Part model, mm, in its own coordinate system. Coordinates: 2 decimals unless noted, no trailing zeros. Loops run counter-clockwise (first coordinate to the right, second up) from the corner with the lowest first, then second, coordinate; pieces in that order, holes last. Notation, with made-up numbers: (64.25, 6) -> (121.25, 6) arc R32 cw to (121.25, 32) -> close; hole circle Ø7 at (69.5, 79.5). An arc over 180 degrees is marked (long way). Use one line per item in the form item = value. Start each with the question number.
(1) Band-saw the part on B-B on x = -126.5. Give the cut face in (y, z), then the cut area to 4 significant figures.
(2) Band-saw the part on A-A on y = -0.6. Give the cut face in (x, z).
(3) Drill centre line: L1, parallel to Z at x = 372.5, y = -0.9. Where is it in solid material? Low to high. Write a range as [from, to].
(4) Pin check, flat tips, straight feed: P1, Ø12, axis at x = -527, z = -2, coming from the +Y side; P2, Ø1.6, axis at x = -306, y = -0.5, coming from the +Z side; P3, Ø1.5, axis at x = -113.5, z = 27.5, coming from the +Y side. Stop position of each tip, or through.
```python
from build123d import *

# Parameters (mm, degrees)
F0_W     = 1380
F0_H     = 60
F1_DEPTH = 3
F2_W     = 1380
F2_H     = 5
F3_DEPTH = 1.5
F4_R     = 2


with BuildPart() as f1:
    # F0 (on Front) → F1 (new body)
    with BuildSketch(Plane.XZ):
        Rectangle(F0_W, F0_H)
    extrude(amount=F1_DEPTH)

    # F2 (on face) → F3 (cut)
    with BuildSketch(Plane(origin=(0, 0, 0), x_dir=(-1, 0, 0), z_dir=(0, 1, 0))):
        with Locations((0, 27.5)):
            Rectangle(F2_W, F2_H)
    extrude(amount=-F3_DEPTH, mode=Mode.SUBTRACT)

    # F4
    f4_edges = [f1.edges().sort_by_distance(p)[0] for p in [
        (690, -2.25, 30),
        (690, -1.5, -30),
        (-690, -2.25, 30),
        (-690, -1.5, -30),
    ]]
    fillet(f4_edges, radius=F4_R)


solid = f1.part
```
A:
q1.outline = (-3, -30) -> (0, -30) -> (0, 25) -> (-1.5, 25) -> (-1.5, 30) -> (-3, 30) -> close
q1.area = 172.5 mm²
q2.outline = (-690, -28) arc R2 ccw to (-688, -30) -> (688, -30) arc R2 ccw to (690, -28) -> (690, 25) -> (-690, 25) -> close
q3.L1 = [-30, 25]
q4.P1 = 0
q4.P2 = 25
q4.P3 = -1.5
